```python
from build123d import *

# Parameters (mm, degrees)
SKETCH1_W           = 7.62
SKETCH1_H           = 18.8214
BOSS_EXTRUDE1_DEPTH = 15.6718
SKETCH2_R           = 0.9906
BOSS_EXTRUDE2_DEPTH = 0.9652
SKETCH3_R           = 3.175
BOSS_EXTRUDE3_DEPTH = 1.4986
SKETCH4_R           = 1.75
BOSS_EXTRUDE4_DEPTH = 2.6924


with BuildPart() as part:
    # Sketch1 → Boss-Extrude1 (new body)
    with BuildSketch(Plane(origin=(0, 0, 0), x_dir=(1, 0, 0), z_dir=(0, 1, 0))):
        with Locations((3.81, 9.4107)):
            Rectangle(SKETCH1_W, SKETCH1_H)
    extrude(amount=BOSS_EXTRUDE1_DEPTH)

    # Sketch2 → Boss-Extrude2 (add)
    # profile 1 of 2: a face of its own
    with BuildSketch(Plane(origin=(0, 11.3284, 0), x_dir=(-1, 0, 0), z_dir=(0, -1, 0))):
        Polygon((0, 0), (-7.62, 0), (-7.62, -3.8735), (-5.08, -3.8735), (-2.54, -3.8735), (0, -3.8735), align=None)
        with Locations(Location((-3.81, -1.7653, 0), (0, 0, 90))):
            Circle(SKETCH2_R, mode=Mode.SUBTRACT)
    # profile 2 of 2: a face of its own
    with BuildSketch(Plane(origin=(0, 11.3284, 0), x_dir=(-1, 0, 0), z_dir=(0, -1, 0))):
        Polygon((-7.62, 18.8214), (0, 18.8214), (0, 22.6949), (-2.54, 22.6949), (-5.08, 22.6949), (-7.62, 22.6949), align=None)
        with Locations(Location((-3.81, 20.5867, 0), (0, 0, 90))):
            Circle(SKETCH2_R, mode=Mode.SUBTRACT)
    extrude(amount=-BOSS_EXTRUDE2_DEPTH)

    # Sketch3 → Boss-Extrude3 (add)
    with BuildSketch(Plane(origin=(0, 15.6718, 0), x_dir=(1, 0, 0), z_dir=(0, 1, 0))):
        with Locations(Location((3.81, 14.8463, 0), (0, 0, 90))):
            Circle(SKETCH3_R)
    extrude(amount=BOSS_EXTRUDE3_DEPTH)

    # Sketch4 → Boss-Extrude4 (add)
    with BuildSketch(Plane(origin=(0, 17.1704, 0), x_dir=(1, 0, 0), z_dir=(0, 1, 0))):
        with Locations(Location((3.81, 14.8463, 0), (0, 0, 270))):
            Circle(SKETCH4_R)
    extrude(amount=BOSS_EXTRUDE4_DEPTH)


solid = part.part
```
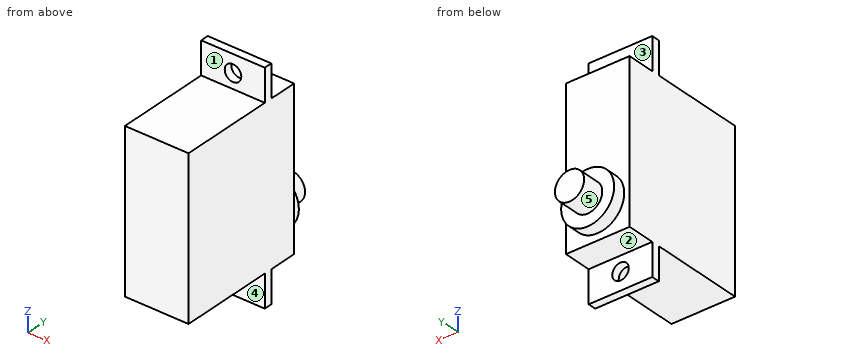
Here's how the part is built. I have some questions about the finished solid (model axes, mm). Face numbers are marked on the shaded views. A direction names the side the tool comes from. Give positions to 0.01 mm unless a question says otherwise; leave off trailing zeros. Write each loop counter-clockwise with the first axis right and the second up, starting at its lowest first coordinate (ties: lowest second). Pieces come first, ordered by that corner, then holes. Notation, with made-up numbers: M 13,79.25 L 19,79.25 A35 cw 19,115.25 Z; hole C 40,79.25 d1. An arc over 180 degrees is marked long. Put each result on its own line as item: value. Start each with the question number.
Item 1: I need wall thicknesses on L1, parallel to Z at x = 2.5, y = 13.25; L2, parallel to Y at x = 3.25, z = -21.5; L3, parallel to Y at x = 7.25, z = -12.75. Which ranges of each line are inside material? Lowest first, please. Write a range as from..to.
Item 2: If we section it at A-A, the plane x = 3.81: Write out the boundary of the cut face in (y, z), then the cut area to 3 significant figures.
Item 3: If we section it at B-B, the plane z = -20.25: Write out the boundary of the cut face in (x, y), then the cut area to 3 significant figures.
Item 4: Will these pins go through, and if not, where does the flat tip stop? pin 1 (1.2 mm diameter, centred on x = 3, z = -21.5, fed in from -Y); pin 2 (2.5 mm diameter, centred on x = 3, y = 13.5, fed in from +Z); pin 3 (2.5 mm diameter, centred on x = 5.5, y = 8.5, fed in from -Z); pin 4 (4 mm diameter, centred on x = 2, y = 2.5, fed in from +Z).
Item 5: On a 3-axis mill with a long thin cutter (end or side, diameter ignored), from which of +Z, -Z, +X, -X, +Y, -Y can I reach the whole of each face in a straight line? I mean the marked faces 1, 2, 3, 4 and 5. Say none if no direction works.
Item 6: If we section it at C-C, the plane z = -15.25: Write out the boundary of the cut face in (x, y), then the cut area to 3 significant figures.
Item 7: If we section it at D-D, the plane y = 10: Write out the boundary of the cut face in (x, z).
Values:
1. L1: -18.82..0
1. L2: 11.33..12.29
1. L3: 0..15.67
2. outline: M 0,-18.82 L 11.33,-18.82 L 11.33,-19.6 L 12.29,-19.6 L 12.29,-18.82 L 15.67,-18.82 L 15.67,-18.02 L 17.17,-18.02 L 17.17,-16.6 L 19.86,-16.6 L 19.86,-13.1 L 17.17,-13.1 L 17.17,-11.67 L 15.67,-11.67 L 15.67,0 L 12.29,0 L 12.29,0.77 L 11.33,0.77 L 11.33,0 L 0,0 Z; M 11.33,-22.69 L 12.29,-22.69 L 12.29,-21.58 L 11.33,-21.58 Z; M 11.33,2.76 L 12.29,2.76 L 12.29,3.87 L 11.33,3.87 Z
2. area: 318 mm²
3. outline: M 0,11.33 L 2.88,11.33 L 2.88,12.29 L 0,12.29 Z; M 4.74,11.33 L 7.62,11.33 L 7.62,12.29 L 4.74,12.29 Z
3. area: 5.56 mm²
4. pin 1: y = 11.33
4. pin 2: z = 3.87
4. pin 3: z = -18.82
4. pin 4: z = 0
5. face 1: +Z, +X, -X, -Y
5. face 2: -Z, +X, -X, +Y
5. face 3: +Z, +X, -X, +Y
5. face 4: -Z, +X, -X, -Y
5. face 5: +Y
6. outline: M 0,0 L 7.62,0 L 7.62,15.67 L 6.96,15.67 L 6.96,17.17 L 5.51,17.17 L 5.51,19.86 L 2.11,19.86 L 2.11,17.17 L 0.66,17.17 L 0.66,15.67 L 0,15.67 Z
6. area: 138 mm²
7. outline: M 0,-18.82 L 7.62,-18.82 L 7.62,0 L 0,0 Z
